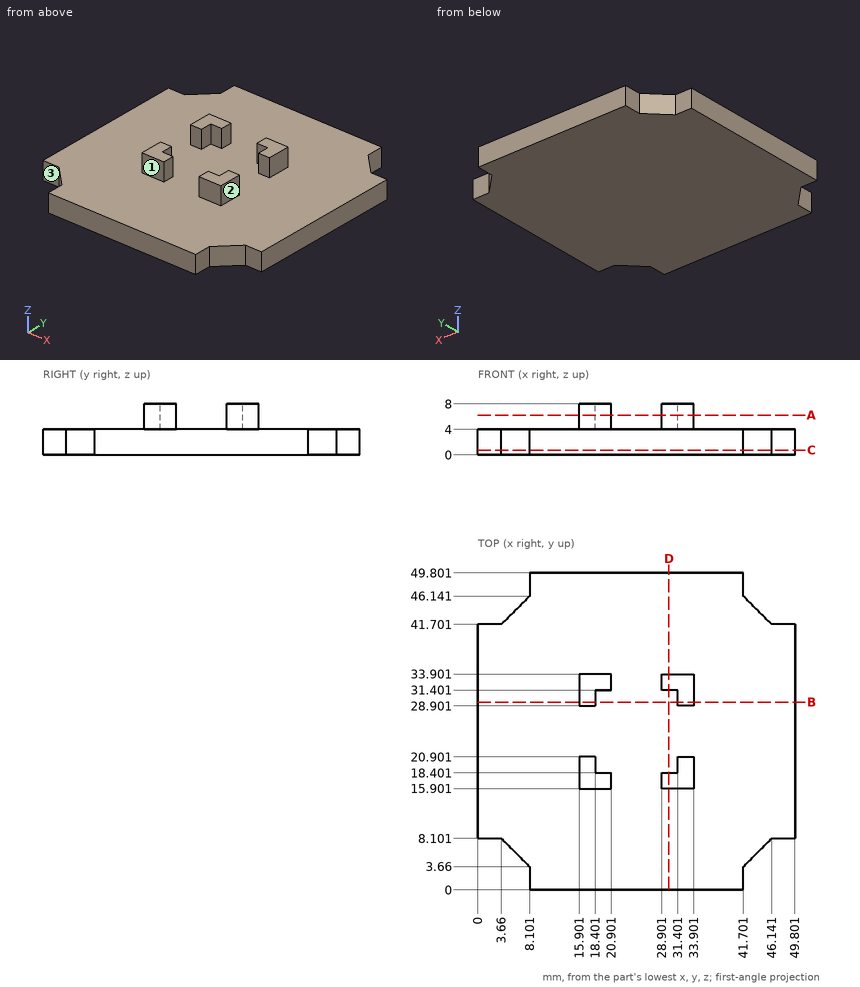
Could you check a few things on this drawing? It's one solid part, dimensions in mm from its lowest x, y, z. A direction names the side the tool comes from. Coordinates: 2 decimals unless noted, no trailing zeros. Order: outer loops, then holes, each group sorted by start corner. A loop starts at its lowest first (then second) coordinate and runs counter-clockwise, first axis right, second up. Notation, with made-up numbers: M -22,9 L 30,9 A28 ccw 30,40 Z; hole C 63,29 d7. An arc over 180 degrees is marked long. Use one line per item in the form item = value. Start each with the question number.
1. On a 3-axis mill with a long thin cutter (end or side, diameter ignored), from which of +Z, -Z, +X, -X, +Y, -Y can I reach the whole of each face in a straight line? I mean the marked faces 1, 2 and 3. Say none if no direction works.
2. Suppose I cut it at C-C on z = 0.75. Write out the boundary of the cut face in (x, y), then the cut area to 3 significant figures.
3. Suppose I cut it at B-B on y = 29.5. Write out the boundary of the cut face in (x, z), then the cut area to 3 significant figures.
4. Please list where these lines run through material, in increasing order: line 1 (Y direction, x = 19, z = 7.25); line 2 (Z direction, x = 34.5, y = 41); line 3 (Y direction, x = 8, z = 0.5).
5. For pin 1 (1.8 mm diameter, centred on x = 1.5, z = 2.5, fed in from -Y); pin 2 (1.8 mm diameter, centred on y = 48, z = 1, fed in from +X); pin 3 (3 mm diameter, centred on x = 13.5, y = 17.5, fed in from +Z), each with a flat end and sliding along its axis, tell me the tip position at first contact or that it passes through.
6. Suppose I cut it at A-A on z = 6.25. Write out the boundary of the cut face in (x, y).
Geometry says:
q1.face_1 = +Z, +X, -X, -Y
q1.face_2 = +Z, +X, +Y, -Y
q1.face_3 = +Z, -Z, -X, -Y
q2.outline = M 0,8.1 L 3.66,8.1 L 8.1,3.66 L 8.1,0 L 41.7,0 L 41.7,3.66 L 46.14,8.1 L 49.8,8.1 L 49.8,41.7 L 46.14,41.7 L 41.7,46.14 L 41.7,49.8 L 8.1,49.8 L 8.1,46.14 L 3.66,41.7 L 0,41.7 Z
q2.area = 2,260 mm^2
q3.outline = M 0,0 L 49.8,0 L 49.8,4 L 33.9,4 L 33.9,8 L 31.4,8 L 31.4,4 L 18.4,4 L 18.4,8 L 15.9,8 L 15.9,4 L 0,4 Z
q3.area = 219 mm^2
q4.line_1 = 15.9 to 18.4, 31.4 to 33.9
q4.line_2 = 0 to 4
q4.line_3 = 3.76 to 46.04
q5.pin_1 = 8.1
q5.pin_2 = 41.7
q5.pin_3 = 4
q6.outline = M 15.9,15.9 L 20.9,15.9 L 20.9,18.4 L 18.4,18.4 L 18.4,20.9 L 15.9,20.9 Z; M 15.9,28.9 L 18.4,28.9 L 18.4,31.4 L 20.9,31.4 L 20.9,33.9 L 15.9,33.9 Z; M 28.9,15.9 L 33.9,15.9 L 33.9,20.9 L 31.4,20.9 L 31.4,18.4 L 28.9,18.4 Z; M 28.9,31.4 L 31.4,31.4 L 31.4,28.9 L 33.9,28.9 L 33.9,33.9 L 28.9,33.9 Z
